Input: part model. Units: mm. Frame: model coordinates. A direction names the side the tool comes from. Round coordinates to 2 decimals unless told otherwise and drop trailing zeros. Loops run counter-clockwise (first coordinate to the right, second up) from the corner with the lowest first, then second, coordinate; pieces in that order, holes last. Notation, with made-up numbers: (83.25, 7.5) -> (89.25, 7.5) arc R5 cw to (89.25, 12.5) -> close; hole circle Ø10 at (24, 66). An arc over 180 degrees is marked (long way). Answer in a Markdown table with one row per item. Add a question column.
Q1. Section C-C, the plane x = 95. Output: boundary loops of the cut face in (y, z), and give its area (3 significant figures).
Q2. Section D-D, the plane x = -83. Output: boundary loops of the cut face in (y, z), and give its area (3 significant figures).
Q3. Pin query (flat end, axial travel): pin 1 (5 mm diameter, centred on x = -105, y = -0.5, fed in from -Z); pin 2 (1.5 mm diameter, centred on x = -10, y = 1.5, fed in from -Z); pin 3 (2 mm diameter, centred on x = 14, z = 3, fed in from +Y). Return the tip coordinate at first contact, or that it passes through.
Q4. Reachability of faces 3 (the face through (-6, -1.668, 2)), 4 (the face through (-4, 3.332, 2)), 5 (the face through (99.62, -1.08, 1.97)), 6 (the face through (-100.38, -1.08, 1.23)), 7 (the face through (-7, 1, 4)) from +Z, -Z, +X, -X, +Y, -Y: full face, straight path, thin tool, end or side. Return the list, or none.
Q5. Section A-A, the plane x = -105. Output: boundary loops of the cut face in (y, z), and give its area (3 significant figures).
Q6. Ray query, L1, parallel to X at y = 1, z = 3.25; L2, parallel to X at y = 4.5, z = 3.05; L3, parallel to Y at x = 95, z = 2.3. Return the intervals inside material, ascending. Write a range as from..to.
Q7. Mould query, pull axis X, two halves, no side actions, for faces 1 (the face through (-7, 1, 0)), 2 (the face through (-114, 1, 2)). Classes: pulls with the +X half, pulls with the -X half, needs draft (parallel to the pull), parting line crosses it, or undercut.
Q8. Section B-B, the plane z = 3.4. Output: boundary loops of the cut face in (x, y), and give its area (3 significant figures).
```python
from build123d import *

# Parameters (mm, degrees)
SKETCH_1_R          = 3
SKETCH_1_R_2        = 5
EXTRUDE_1_DEPTH     = 4
SKETCH_1_3_R        = 5
CUT_EXTRUDE_1_DEPTH = 2.5


with BuildPart() as part:
    # 草图1 → 凸台-拉伸1 (new body)
    with BuildSketch(Plane.XY):
        with BuildLine():
            Line((-95, -1.668248682), (85, -1.668248682))
            Line((85, -1.668248682), (87, -3.291354308))
            ThreePointArc((87, -3.291354308), (104, 0.831751318), (87, 4.954856943))
            ThreePointArc((87, 4.954856943), (86.004567475, 4.137676062), (85, 3.331751318))
            Line((85, 3.331751318), (-95, 3.331751318))
            ThreePointArc((-95, 3.331751318), (-96.007924928, 4.133538989), (-97, 4.954856943))
            ThreePointArc((-97, 4.954856943), (-114, 0.831751318), (-97, -3.291354308))
            ThreePointArc((-97, -3.291354308), (-96.287873429, -2.125082216), (-95, -1.668248682))
        make_face()
        with Locations((-105, 0.831751318)):
            Circle(SKETCH_1_R, mode=Mode.SUBTRACT)
        with Locations((95, 0.831751318)):
            Circle(SKETCH_1_R_2, mode=Mode.SUBTRACT)
    extrude(amount=EXTRUDE_1_DEPTH)

    # 草图1<3> → 切除-拉伸1 (cut)
    with BuildSketch(Plane.XY):
        with Locations((-105, 0.831751318)):
            Circle(SKETCH_1_3_R)
    extrude(amount=CUT_EXTRUDE_1_DEPTH, mode=Mode.SUBTRACT)


solid = part.part
```
Answer block:
| question | item | result |
|---|---|---|
| 1 | outline | (-8.17, 0) -> (-4.17, 0) -> (-4.17, 4) -> (-8.17, 4) -> close; (5.83, 0) -> (9.83, 0) -> (9.83, 4) -> (5.83, 4) -> close |
| 1 | area | 32.0 mm^2 |
| 2 | outline | (-1.67, 0) -> (3.33, 0) -> (3.33, 4) -> (-1.67, 4) -> close |
| 2 | area | 20.0 mm^2 |
| 3 | pin 1 | z = 2.5 |
| 3 | pin 2 | z = 0 |
| 3 | pin 3 | y = 3.33 |
| 4 | face 3 | +Z, -Z, -Y |
| 4 | face 4 | +Z, -Z, +Y |
| 4 | face 5 | +Z, -Z |
| 4 | face 6 | -Z |
| 4 | face 7 | +Z, +X, -X, +Y, -Y |
| 5 | outline | (-8.17, 0) -> (-4.17, 0) -> (-4.17, 2.5) -> (-2.17, 2.5) -> (-2.17, 4) -> (-8.17, 4) -> close; (3.83, 2.5) -> (5.83, 2.5) -> (5.83, 0) -> (9.83, 0) -> (9.83, 4) -> (3.83, 4) -> close |
| 5 | area | 38.0 mm^2 |
| 6 | L1 | -114..-108, -102..90, 100..104 |
| 6 | L2 | -113.22..-96.46, 86.45..91.6, 98.4..103.22 |
| 6 | L3 | -8.17..-4.17, 5.83..9.83 |
| 7 | face 1 | needs draft |
| 7 | face 2 | undercut |
| 8 | outline | (-97, -3.29) arc R2.04 cw to (-95, -1.67) -> (85, -1.67) -> (87, -3.29) arc R9 ccw (long way) to (87, 4.95) arc R114.42 cw to (85, 3.33) -> (-95, 3.33) arc R65.95 cw to (-97, 4.95) arc R9 ccw (long way) to start; hole circle Ø6 at (-105, 0.83); hole circle Ø10 at (95, 0.83) |
| 8 | area | 1,320 mm^2 |
